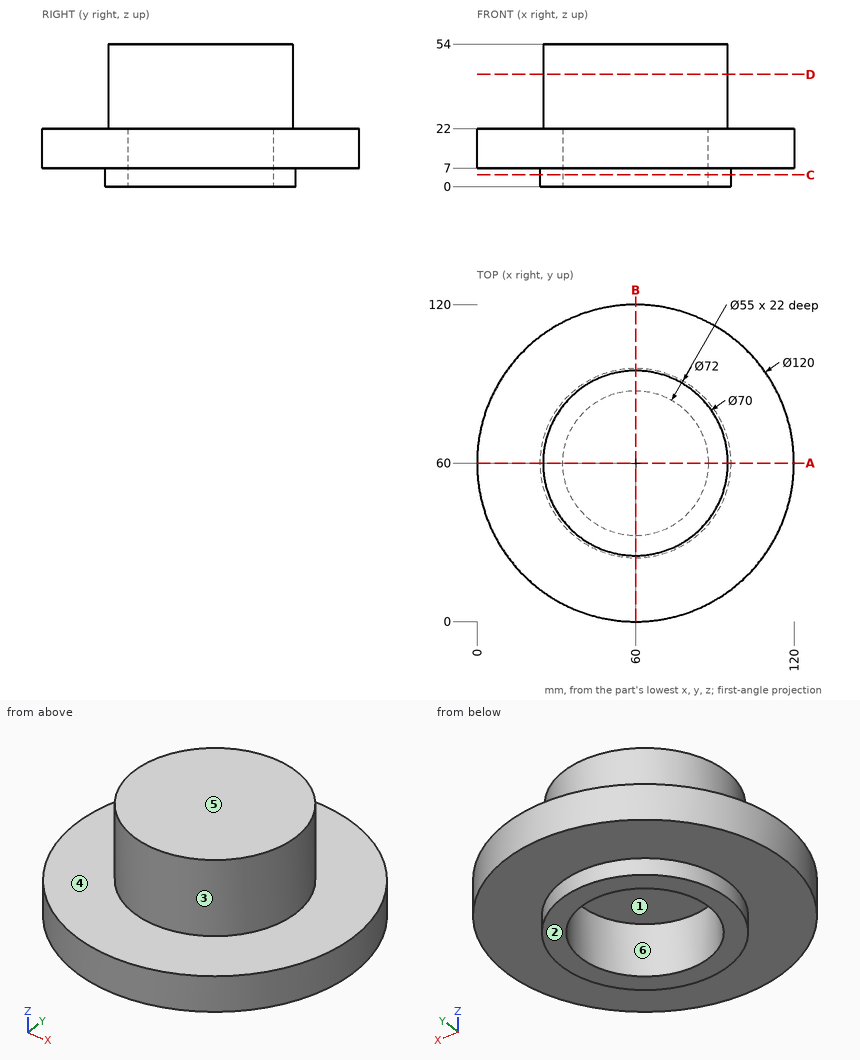
The figure shows three views and two pictorial views of one solid part (mm, origin at its lowest corner). Answer the questions. A direction names the side the tool comes from. Round coordinates to 2 decimals unless told otherwise and drop trailing zeros. Loops run counter-clockwise (first coordinate to the right, second up) from the corner with the lowest first, then second, coordinate; pieces in that order, holes last. Notation, with made-up numbers: M 84.25,10.25 L 91.25,10.25 A28 ccw 91.25,28.25 Z; hole C 35,-30.5 d11. An arc over 180 degrees is marked long. Write each question's results on one line, items separated by ' | '. Start each with the question number.
1) Determine the mould class of the marked faces 1, 2 and 3 for opening direction X: pulls with the +X half, pulls with the -X half, needs draft (parallel to the pull), parting line crosses it, or undercut.
2) Find section C-C on z = 4.5. Write down the section's boundary in (x, y), plus the area to 3 significant figures.
3) Each of these flat-tipped pins is pushed along its axis until it touches: pin 1 (2 mm diameter, centred on y = 52.5, z = 39, fed in from -X); pin 2 (1.5 mm diameter, centred on x = 104, y = 61.5, fed in from +Z); pin 3 (1.5 mm diameter, centred on y = 54.5, z = 40, fed in from +X). Where does it stop, or does it pass through?
4) Straight lines are drawn through the part: probe 1 along Y at (x, z) = (61, 17.5); probe 2 along Z at (x, y) = (73.5, 42); probe 3 along Z at (x, y) = (33.5, 17.5). For each, find the intervals that lie inside material, in ascending order.
5) Find section D-D on z = 42.5. Write down the section's boundary in (x, y), plus the area to 3 significant figures.
6) Find section A-A on y = 60. Write down the section's boundary in (x, z), plus the area to 3 significant figures.
7) Which of the six approach directions +Z, -Z, +X, -X, +Y, -Y give full straight-line access (tool end or side, diameter ignored) to the marked faces 4, 5 and 6?
Final values:
1) face 1: undercut | face 2: needs draft | face 3: parting line crosses it
2) outline: C 60,60 d72; hole C 60,60 d55 | area: 1,700 mm²
3) pin 1: x = 25.61 | pin 2: z = 22 | pin 3: x = 94.68
4) probe 1: 0.01 to 32.52, 87.48 to 119.99 | probe 2: 22 to 54 | probe 3: 7 to 22
5) outline: C 60,60 d70 | area: 3,850 mm²
6) outline: M 0,7 L 24,7 L 24,0 L 32.5,0 L 32.5,22 L 87.5,22 L 87.5,0 L 96,0 L 96,7 L 120,7 L 120,22 L 95,22 L 95,54 L 25,54 L 25,22 L 0,22 Z | area: 3,330 mm²
7) face 4: +Z | face 5: +Z, +X, -X, +Y, -Y | face 6: -Z
